Verification items for the finished model (mm, model axes). A direction names the side the tool comes from. Give positions to 0.01 mm unless a question says otherwise; leave off trailing zeros. Write each loop counter-clockwise with the first axis right and the second up, starting at its lowest first coordinate (ties: lowest second). Pieces come first, ordered by that corner, then holes. Notation, with made-up numbers: (47, -18) - (79, -18) arc R30 ccw to (79, 4) - close; hole circle Ø11 at (84, 31.5). An arc over 180 degrees is marked (long way). Put each result on its own line as item: value.
from build123d import *

# Parameters (mm, degrees)
SKETCH_1_W                      = 15
SKETCH_1_H                      = 15
EXTRUDE_1_DEPTH                 = 15
SKETCH_2_W                      = 13
SKETCH_2_H                      = 11
CUT_EXTRUDE_1_DEPTH             = 13
EXTRUDE_START                   = -4.5
EXTRUDE_2_DEPTH                 = 6
SKETCH_5_W                      = 3
SKETCH_5_H                      = 3
EXTRUDE_3_DEPTH                 = 1
CUT_EXTRUDE_3_REACH             = 26.238
CUT_EXTRUDE_4_REACH             = 29.5
CUT_EXTRUDE_5_REACH             = 26.238
CUT_EXTRUDE_5_DIRECTION_2_REACH = 26.238
FILLET_1_R                      = 0.1
FILLET_2_R                      = 0.2
EXTRUDE_4_DEPTH                 = 3
EXTRUDE_4_DEPTH_BACK            = 3
CUT_EXTRUDE_6_DEPTH             = 15
FILLET_3_R                      = 0.1


with BuildPart() as part:
    # Sketch 1 → Extrude 1 (new body)
    with BuildSketch(Plane.XY):
        with Locations((0, 7.5)):
            Rectangle(SKETCH_1_W, SKETCH_1_H)
    extrude(amount=-EXTRUDE_1_DEPTH)

    # Sketch 2 → Cut-Extrude 1 (cut)
    with BuildSketch(Plane.ZY.offset(7.5)):
        with Locations((-6.5, 7.5)):
            Rectangle(SKETCH_2_W, SKETCH_2_H)
    extrude(amount=-CUT_EXTRUDE_1_DEPTH, mode=Mode.SUBTRACT)



with BuildPart() as body_2:
    # Sketch 4 → Extrude 2 (new body)
    with BuildSketch(Plane.XY.offset(EXTRUDE_START)):
        with BuildLine():
            Line((-1.5, 15.677124344), (1.5, 15.677124344))
            ThreePointArc((1.5, 15.677124344), (1.780042303, 16.088161527), (1.95, 16.555590279))
            Line((1.95, 16.555590279), (1.95, 17.5))
            Line((1.95, 17.5), (-1.95, 17.5))
            Line((-1.95, 17.5), (-1.95, 16.555590279))
            ThreePointArc((-1.95, 16.555590279), (-1.780042303, 16.088161527), (-1.5, 15.677124344))
        make_face()
    extrude(amount=-EXTRUDE_2_DEPTH)


with BuildPart() as part_1:
    add(part.part)

    add(body_2.part)  # Extrude 3 merges body 2
    # Sketch 5 → Extrude 3 (add)
    with BuildSketch(Plane(origin=(0, 15, 0), x_dir=(-1, 0, 0), z_dir=(0, 1, 0))):
        with Locations((0, -7.5)):
            Rectangle(SKETCH_5_W, SKETCH_5_H)
    extrude(amount=EXTRUDE_3_DEPTH)

    # Sketch 6 → Cut-Extrude 3 (cut, up to next)
    with BuildSketch(Plane(origin=(0, 0, -15), x_dir=(-1, 0, 0), z_dir=(0, 0, -1)), mode=Mode.PRIVATE) as cut_extrude_3_sk1:
        with BuildLine():
            Line((-1.5, 6.177124344), (-1.5, 4))
            Line((-1.5, 4), (1.5, 4))
            Line((1.5, 4), (1.5, 6.177124344))
            ThreePointArc((1.5, 6.177124344), (2, 7.5), (1.5, 8.822875656))
            Line((1.5, 8.822875656), (1.5, 11))
            Line((1.5, 11), (-1.5, 11))
            Line((-1.5, 11), (-1.5, 8.822875656))
            ThreePointArc((-1.5, 8.822875656), (-2, 7.5), (-1.5, 6.177124344))
        make_face()
    cut_extrude_3_tool1 = extrude(cut_extrude_3_sk1.sketch, amount=-CUT_EXTRUDE_3_REACH, mode=Mode.PRIVATE) & part_1.part
    add(cut_extrude_3_tool1.solids().sort_by_distance((0, 7.5, -15))[0], mode=Mode.SUBTRACT)

    # Sketch 7 → Cut-Extrude 4 (cut, up to next)
    with BuildSketch(Plane(origin=(7.5, 0, 0), x_dir=(0, 0, -1), z_dir=(1, 0, 0)), mode=Mode.PRIVATE) as cut_extrude_4_sk1:
        with BuildLine():
            Line((6, 6.177124344), (6, 4))
            Line((6, 4), (9, 4))
            Line((9, 4), (9, 6.177124344))
            ThreePointArc((9, 6.177124344), (9.5, 7.5), (9, 8.822875656))
            Line((9, 8.822875656), (9, 11))
            Line((9, 11), (6, 11))
            Line((6, 11), (6, 8.822875656))
            ThreePointArc((6, 8.822875656), (5.5, 7.5), (6, 6.177124344))
        make_face()
    cut_extrude_4_tool1 = extrude(cut_extrude_4_sk1.sketch, amount=-CUT_EXTRUDE_4_REACH, mode=Mode.PRIVATE) & part_1.part
    add(cut_extrude_4_tool1.solids().sort_by_distance((7.5, 7.5, -7.5))[0], mode=Mode.SUBTRACT)

    # Sketch 8 → Cut-Extrude 5 (cut, up to next)
    with BuildSketch(Plane(origin=(0, 0, 0), x_dir=(0, 0, -1), z_dir=(1, 0, 0)), mode=Mode.PRIVATE) as cut_extrude_5_sk1:
        with BuildLine():
            Line((5.55, 17.5), (5.55, 16.555590279))
            ThreePointArc((5.55, 16.555590279), (5.719957697, 16.088161527), (6, 15.677124344))
            Line((6, 15.677124344), (4.5, 15.677124344))
            Line((4.5, 15.677124344), (4.5, 17.5))
            Line((4.5, 17.5), (5.55, 17.5))
        make_face()
    cut_extrude_5_tool1 = extrude(cut_extrude_5_sk1.sketch, amount=-CUT_EXTRUDE_5_REACH, mode=Mode.PRIVATE) & part_1.part
    # Sketch 8 → Cut-Extrude 5 (cut, up to next)
    with BuildSketch(Plane(origin=(0, 0, 0), x_dir=(0, 0, -1), z_dir=(1, 0, 0)), mode=Mode.PRIVATE) as cut_extrude_5_sk2:
        with BuildLine():
            Line((10.5, 17.5), (9.45, 17.5))
            Line((9.45, 17.5), (9.45, 16.555590279))
            ThreePointArc((9.45, 16.555590279), (9.280042303, 16.088161527), (9, 15.677124344))
            Line((9, 15.677124344), (10.5, 15.677124344))
            Line((10.5, 15.677124344), (10.5, 17.5))
        make_face()
    cut_extrude_5_tool2 = extrude(cut_extrude_5_sk2.sketch, amount=-CUT_EXTRUDE_5_REACH, mode=Mode.PRIVATE) & part_1.part
    add(cut_extrude_5_tool1.solids().sort_by_distance((0, 16.539049, -5.075076))[0], mode=Mode.SUBTRACT)
    add(cut_extrude_5_tool2.solids().sort_by_distance((0, 16.539049, -9.924924))[0], mode=Mode.SUBTRACT)

    # Sketch 8 → Cut-Extrude 5 direction 2 (cut, up to next)
    with BuildSketch(Plane(origin=(0, 0, 0), x_dir=(0, 0, -1), z_dir=(1, 0, 0)), mode=Mode.PRIVATE) as cut_extrude_5_direction_2_sk1:
        with BuildLine():
            Line((5.55, 17.5), (5.55, 16.555590279))
            ThreePointArc((5.55, 16.555590279), (5.719957697, 16.088161527), (6, 15.677124344))
            Line((6, 15.677124344), (4.5, 15.677124344))
            Line((4.5, 15.677124344), (4.5, 17.5))
            Line((4.5, 17.5), (5.55, 17.5))
        make_face()
    cut_extrude_5_direction_2_tool1 = extrude(cut_extrude_5_direction_2_sk1.sketch, amount=CUT_EXTRUDE_5_DIRECTION_2_REACH, mode=Mode.PRIVATE) & part_1.part
    # Sketch 8 → Cut-Extrude 5 direction 2 (cut, up to next)
    with BuildSketch(Plane(origin=(0, 0, 0), x_dir=(0, 0, -1), z_dir=(1, 0, 0)), mode=Mode.PRIVATE) as cut_extrude_5_direction_2_sk2:
        with BuildLine():
            Line((10.5, 17.5), (9.45, 17.5))
            Line((9.45, 17.5), (9.45, 16.555590279))
            ThreePointArc((9.45, 16.555590279), (9.280042303, 16.088161527), (9, 15.677124344))
            Line((9, 15.677124344), (10.5, 15.677124344))
            Line((10.5, 15.677124344), (10.5, 17.5))
        make_face()
    cut_extrude_5_direction_2_tool2 = extrude(cut_extrude_5_direction_2_sk2.sketch, amount=CUT_EXTRUDE_5_DIRECTION_2_REACH, mode=Mode.PRIVATE) & part_1.part
    add(cut_extrude_5_direction_2_tool1.solids().sort_by_distance((0, 16.539049, -5.075076))[0], mode=Mode.SUBTRACT)
    add(cut_extrude_5_direction_2_tool2.solids().sort_by_distance((0, 16.539049, -9.924924))[0], mode=Mode.SUBTRACT)

    # Fillet 1
    fillet_1_edges = [part_1.edges().sort_by_distance(p)[0] for p in [
        (0, 17.5, -5.55),
        (1.95, 17.5, -7.5),
        (-1.95, 17.5, -7.5),
        (0, 17.5, -9.45),
    ]]
    fillet(fillet_1_edges, radius=FILLET_1_R)

    # Fillet 2
    fillet_2_edges = [part_1.edges().sort_by_distance(p)[0] for p in [
        (0, 0, 0),
        (7.5, 0, -7.5),
        (0, 0, -15),
        (-7.5, 0, -7.5),
        (7.5, 7.5, -15),
        (0, 15, -15),
        (-7.5, 15, -7.5),
        (-7.5, 7.5, -15),
        (-7.5, 1, 0),
        (7.5, 7.5, 0),
        (7.5, 15, -7.5),
        (0, 15, 0),
    ]]
    fillet(fillet_2_edges, radius=FILLET_2_R)

    # Sketch 9 → Extrude 4 (add, two sides: drawn at the far end of the back side and taken through both)
    with BuildSketch(Plane(origin=(0, 0, 0), x_dir=(0, 0, -1), z_dir=(1, 0, 0)).offset(-EXTRUDE_4_DEPTH_BACK)):
        with BuildLine():
            Line((6, 0), (9, 0))
            Line((9, 0), (9, -0.677124344))
            ThreePointArc((9, -0.677124344), (9.280042303, -1.088161527), (9.45, -1.555590279))
            Line((9.45, -1.555590279), (9.45, -2.5))
            Line((9.45, -2.5), (5.55, -2.5))
            Line((5.55, -2.5), (5.55, -1.555590279))
            ThreePointArc((5.55, -1.555590279), (5.719957697, -1.088161527), (6, -0.677124344))
            Line((6, -0.677124344), (6, 0))
        make_face()
    extrude(amount=EXTRUDE_4_DEPTH + EXTRUDE_4_DEPTH_BACK)

    # Sketch 10 → Cut-Extrude 6 (cut)
    with BuildSketch(Plane.XY):
        with BuildLine():
            Line((-1.95, -2.5), (-1.95, -1.555590279))
            ThreePointArc((-1.95, -1.555590279), (-1.780042303, -1.088161527), (-1.5, -0.677124344))
            Line((-1.5, -0.677124344), (-1.5, 0))
            Line((-1.5, 0), (-3, 0))
            Line((-3, 0), (-3, -2.5))
            Line((-3, -2.5), (-1.95, -2.5))
        make_face()
        with BuildLine():
            Line((1.5, 0), (1.5, -0.677124344))
            ThreePointArc((1.5, -0.677124344), (1.780042303, -1.088161527), (1.95, -1.555590279))
            Line((1.95, -1.555590279), (1.95, -2.5))
            Line((1.95, -2.5), (3, -2.5))
            Line((3, -2.5), (3, 0))
            Line((3, 0), (1.5, 0))
        make_face()
    extrude(amount=-CUT_EXTRUDE_6_DEPTH, mode=Mode.SUBTRACT)

    # Fillet 3
    fillet_3_edges = [part_1.edges().sort_by_distance(p)[0] for p in [
        (0, -2.5, -9.45),
        (0, -2.5, -5.55),
        (-1.95, -2.5, -7.5),
        (1.95, -2.5, -7.5),
    ]]
    fillet(fillet_3_edges, radius=FILLET_3_R)


solid = part_1.part
Q1. Section check A-A, the plane y = 4.5. Record the cut outline in (x, z).
Answers follow:
outline: (-7.5, -14.8) arc R0.2 ccw to (-7.3, -15) - (-1.5, -15) - (-1.5, -13) - (-7.5, -13) - close; (1.5, -15) - (7.3, -15) arc R0.2 ccw to (7.5, -14.8) - (7.5, -9) - (5.5, -9) - (5.5, -13) - (1.5, -13) - close; (5.5, -6) - (7.5, -6) - (7.5, -0.2) arc R0.2 ccw to (7.3, 0) - (5.5, 0) - close
Q2. Set-up check for faces 1 (the face through (0, 4, -14)), 2 (the face through (5.5, 8, -5)), 3 (the face through (7, 10, -6)), 4 (the face through (0, -2, -9.45)): record each of +Z, -Z, +X, -X, +Y, -Y from which the full face is reachable in a straight line by a thin tool's end or side.
Answers follow:
face 1: +Z, -Z
face 2: +Z, -X
face 3: +X, -X
face 4: -Z, +X, -X, -Y
Q3. Section check C-C, the plane x = 5. Record the cut outline in (y, z), plus the area to 3 significant figures.
Answers follow:
outline: (0, -14.8) arc R0.2 ccw to (0.2, -15) - (14.8, -15) arc R0.2 ccw to (15, -14.8) - (15, -0.2) arc R0.2 ccw to (14.8, 0) - (13, 0) - (13, -13) - (2, -13) - (2, 0) - (0.2, 0) arc R0.2 ccw to (0, -0.2) - close
area: 82.0 mm2
Q4. Section check D-D, the plane z = -12. Record the cut outline in (x, y), plus the area to 3 significant figures.
Answers follow:
outline: (-7.5, 0.2) arc R0.2 ccw to (-7.3, 0) - (7.3, 0) arc R0.2 ccw to (7.5, 0.2) - (7.5, 14.8) arc R0.2 ccw to (7.3, 15) - (-7.3, 15) arc R0.2 ccw to (-7.5, 14.8) - (-7.5, 13) - (5.5, 13) - (5.5, 2) - (-7.5, 2) - close
area: 82.0 mm2
Q5. Go/stop test with flat-tipped pins: pin 1 Ø3 at (x, z) = (-5, -7) entering from -Y; pin 2 Ø0.9 at (x, y) = (0, -2) entering from -Z; pin 3 Ø0.7 at (y, z) = (15.5, -7) entering from +X. Record where each tip stops, or that it passes through.
Answers follow:
pin 1: stops at y = 0
pin 2: stops at z = -9.45
pin 3: stops at x = 1.64
Q6. Section check B-B, the plane z = -14. Record the cut outline in (x, y).
Answers follow:
outline: (-7.5, 0.2) arc R0.2 ccw to (-7.3, 0) - (7.3, 0) arc R0.2 ccw to (7.5, 0.2) - (7.5, 14.8) arc R0.2 ccw to (7.3, 15) - (-7.3, 15) arc R0.2 ccw to (-7.5, 14.8) - close; hole (-1.5, 4) - (1.5, 4) - (1.5, 6.18) arc R2 ccw to (1.5, 8.82) - (1.5, 11) - (-1.5, 11) - (-1.5, 8.82) arc R2 ccw to (-1.5, 6.18) - close
Q7. Release check for a two-part mould opening along Y. For faces 5 (the face through (7, 4, -7)), 6 (the face through (0, 17, -9.45)) record: released by +Y, released by -Y, zero draft, split by the parting line, or undercut.
Answers follow:
face 5: undercut
face 6: zero draft
Q8. Scan lines: line 1 along Y through (x, z) = (-2.5, -11.5); line 2 along Y through (x, z) = (0.5, -8.75); line 3 along X through (y, z) = (8.75, -5.25). Record each from-to range of solid material in increasing order.
Answers follow:
line 1: y = 0 to 2, 13 to 15
line 2: y = -2.5 to 2, 13 to 17.5
line 3: x = 5.5 to 7.5
